from build123d import *

# Parameters (mm, degrees)
SKETCH3_W          = 229.663439326
SKETCH3_H          = 40
CUT_EXTRUDE1_DEPTH = 30


with BuildPart() as part:
    # Sketch1 → Revolve1 (revolve)
    with BuildSketch(Plane.XY):
        Polygon((0, 0), (-45, 0), (-45, 105), (-75, 105), (-75, 130), (-90, 130), (-90, 180), (0, 180), align=None)
    revolve(axis=Axis((0, 209.327847516, 0), (0, -1, 0)))

    # Sketch2 → Cut-Revolve3 (revolve, cut)
    with BuildSketch(Plane.XY):
        Polygon((25, 0), (25, 125), (60, 125), (60, 145), (75, 145), (75, 180), (0, 180), (0, 0), align=None)
    revolve(axis=Axis((0, 180, 0), (0, -1, 0)), mode=Mode.SUBTRACT)

    # Sketch3 → Cut-Extrude1 (cut)
    with BuildSketch(Plane(origin=(0, 180, 0), x_dir=(1, 0, 0), z_dir=(0, 1, 0))):
        Rectangle(SKETCH3_W, SKETCH3_H)
    extrude(amount=-CUT_EXTRUDE1_DEPTH, mode=Mode.SUBTRACT)


solid = part.part
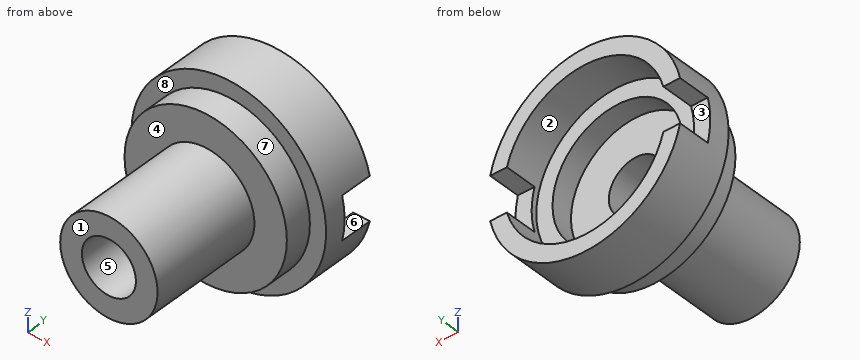
Verification items for the finished model (mm, model axes). Face numbers are marked on the shaded views. A direction names the side the tool comes from. Coordinates: 2 decimals unless noted, no trailing zeros. Order: outer loops, then holes, each group sorted by start corner. A loop starts at its lowest first (then second) coordinate and runs counter-clockwise, first axis right, second up. Notation, with made-up numbers: M 62.5,58.5 L 70.5,58.5 A18 cw 70.5,86.5 Z; hole C -28.5,50 d7. An arc over 180 degrees is marked long. One line per item, written item: value. Start each with the question number.
Item 1: Mould release check, pull along Z, two halves, no side actions. Record for the marked faces 6, 7 and 8: pulls with the +Z half, pulls with the -Z half, needs draft (parallel to the pull), parting line crosses it, or undercut.
Item 2: Sectioned sample at C-C on y = 120. Record the cut outline in (x, z), then the cut area to 3 significant figures.
Item 3: Access from +Z, -Z, +X, -X, +Y, -Y to the whole of each face (thin tool, end or side, straight path). Record for the marked faces 1, 2, 3, 4 and 5.
Item 4: Depth check by flat-ended pin: P1, Ø2, axis at y = 117.5, z = 13.5, coming from the -X side; P2, Ø8, axis at y = 48, z = 45.5, coming from the -X side; P3, Ø12.5, axis at x = -82, y = 160.5, coming from the -Z side; P4, Ø10, axis at x = -30, z = -35.5, coming from the -Y side. Enter the tip coordinate at first touch or a pass-through.
Item 5: Sectioned sample at B-B on x = 0. Record the cut outline in (y, z).
Item 6: Sectioned sample at D-D on x = -56. Record the cut outline in (y, z).
Item 7: Sectioned sample at A-A on z = 0. Record the cut outline in (x, y), then the cut area to 3 significant figures.
Item 8: Thickness scan on probe 1 along Z at (x, y) = (0, 86.5); probe 2 along Y at (x, z) = (-36.5, 20); probe 3 along Y at (x, z) = (-64, -18). Record the ranges inside material, lowest first.
Calculated:
1. face 6: undercut
1. face 7: parting line crosses it
1. face 8: needs draft
2. outline: C 0,0 d150; hole C 0,0 d50
2. area: 15,700 mm^2
3. face 1: +Z, -Z, +X, -X, -Y
3. face 2: +Y
3. face 3: +X, -X, +Y
3. face 4: -Y
3. face 5: +Y, -Y
4. P1: x = -73.95
4. P2: x = -17.4
4. P3: z = -48.6
4. P4: y = 0
5. outline: M 0,-45 L 105,-45 L 105,-75 L 130,-75 L 130,-90 L 180,-90 L 180,-75 L 145,-75 L 145,-60 L 125,-60 L 125,-25 L 0,-25 Z; M 0,25 L 125,25 L 125,60 L 145,60 L 145,75 L 180,75 L 180,90 L 130,90 L 130,75 L 105,75 L 105,45 L 0,45 Z
6. outline: M 105,-49.89 L 130,-49.89 L 130,-70.46 L 180,-70.46 L 180,-49.89 L 145,-49.89 L 145,-21.54 L 125,-21.54 L 125,21.54 L 145,21.54 L 145,49.89 L 180,49.89 L 180,70.46 L 130,70.46 L 130,49.89 L 105,49.89 Z
7. outline: M -90,130 L -75,130 L -75,105 L -45,105 L -45,0 L -25,0 L -25,125 L -60,125 L -60,145 L -75,145 L -75,150 L -90,150 Z; M 25,0 L 45,0 L 45,105 L 75,105 L 75,130 L 90,130 L 90,150 L 75,150 L 75,145 L 60,145 L 60,125 L 25,125 Z
7. area: 7,400 mm^2
8. probe 1: -45 to -25, 25 to 45
8. probe 2: 0 to 125
8. probe 3: 105 to 145
